Input: dimensioned drawing with shaded views. Units: mm. Origin: part minimum x, y, z. Round coordinates to 2 decimals unless told otherwise and drop trailing zeros. Loops run counter-clockwise (first coordinate to the right, second up) from the corner with the lowest first, then second, coordinate; pieces in that order, holes last. Notation, with made-up numbers: (9, -38.5) - (60, -38.5) arc R22 cw to (60, -21.5) - close; hole circle Ø1 at (32.25, 31). An arc over 180 degrees is marked (long way). One line per question, with ' | ' between items. Start each with the question number.
1. Ray query, line 1 (Y direction, x = 16.5, z = 86.5); line 2 (Z direction, x = 202, y = 103). Return the intervals inside material, ascending.
2. Cut plane B-B (z = 123). Return loops of the section in (x, y).
3. Mould query, pull axis Y, two halves, no side actions, for the marked faces 1, 2 and 3. Classes: pulls with the +Y half, pulls with the -Y half, needs draft (parallel to the pull), parting line crosses it, or undercut.
4. Cut plane A-A (y = 203.5). Return loops of the section in (x, z).
5. Cut plane C-C (y = 24.5). Return loops of the section in (x, z), then the cut area to 3 significant figures.
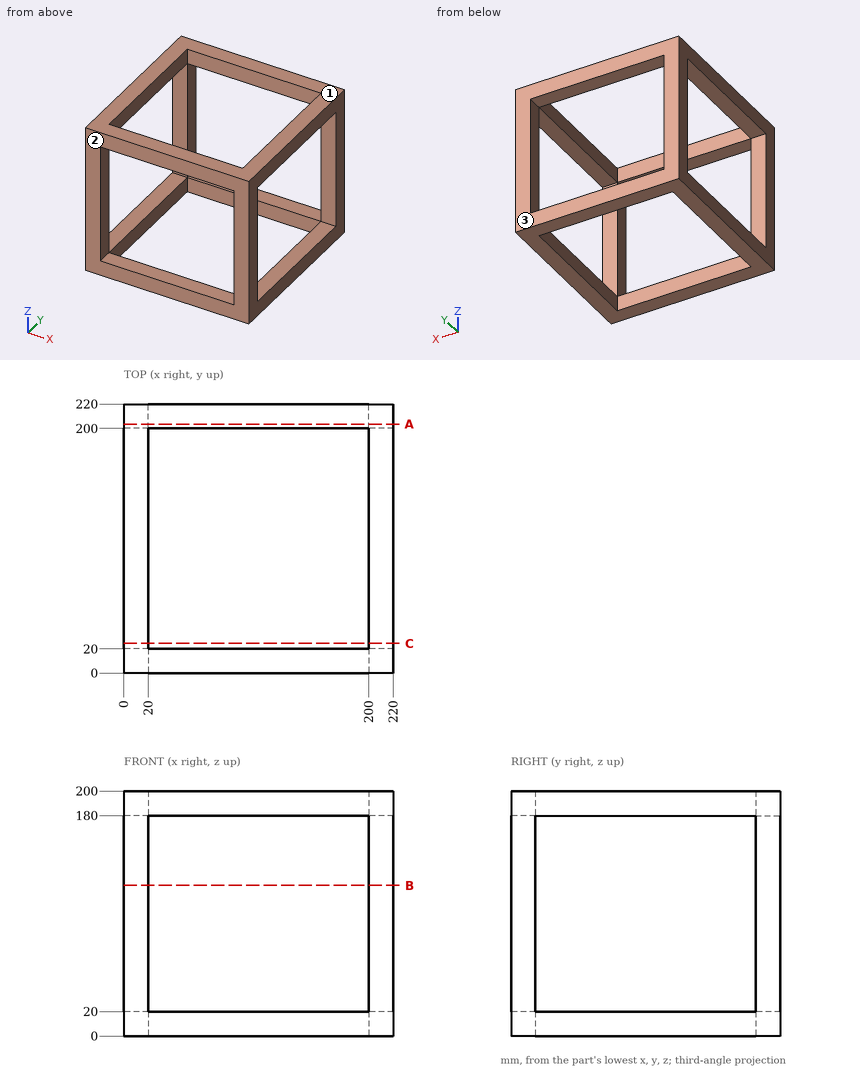
Answers follow:
1) line 1: y = 0 to 20, 200 to 220 | line 2: z = 0 to 20, 180 to 200
2) outline: (0, 0) - (20, 0) - (20, 20) - (0, 20) - close; (0, 200) - (20, 200) - (20, 220) - (0, 220) - close; (200, 0) - (220, 0) - (220, 20) - (200, 20) - close; (200, 200) - (220, 200) - (220, 220) - (200, 220) - close
3) face 1: needs draft | face 2: pulls with the -Y half | face 3: pulls with the +Y half
4) outline: (0, 0) - (220, 0) - (220, 200) - (0, 200) - close; hole (20, 20) - (200, 20) - (200, 180) - (20, 180) - close
5) outline: (0, 0) - (20, 0) - (20, 20) - (0, 20) - close; (0, 180) - (20, 180) - (20, 200) - (0, 200) - close; (200, 0) - (220, 0) - (220, 20) - (200, 20) - close; (200, 180) - (220, 180) - (220, 200) - (200, 200) - close | area: 1,600 mm2
